```python
from build123d import *

# Parameters (mm, degrees)
CYLINDER002_R           = 2
CYLINDER002_DEPTH       = 10
CYLINDER002_PITCH_ANGLE = 90
CYLINDER003_R           = 2
CYLINDER003_DEPTH       = 10
CYLINDER003_PITCH_ANGLE = 90
CYLINDER001_R           = 2
CYLINDER001_DEPTH       = 10
CYLINDER001_PITCH_ANGLE = 90
CYLINDER_R              = 2
CYLINDER_DEPTH          = 10
CYLINDER_PITCH_ANGLE    = 90
BOX012_W                = 10
BOX012_H                = 4.3
BOX012_DEPTH            = 13
BOX011_W                = 10
BOX011_H                = 1.8
BOX011_DEPTH            = 13
BOX007_W                = 10
BOX007_H                = 1.8
BOX007_DEPTH            = 13
BOX009_W                = 10
BOX009_H                = 4.3
BOX009_DEPTH            = 13
BOX008_W                = 10
BOX008_H                = 4.3
BOX008_DEPTH            = 13
BOX010_W                = 10
BOX010_H                = 1.8
BOX010_DEPTH            = 13
BOX006_W                = 10
BOX006_H                = 4.3
BOX006_DEPTH            = 13
BOX005_W                = 10
BOX005_H                = 1.8
BOX005_DEPTH            = 13
BOX002_W                = 10
BOX002_H                = 25
BOX002_DEPTH            = 77.4
BOX004_W                = 10
BOX004_H                = 25
BOX004_DEPTH            = 77.4
BOX001_W                = 10
BOX001_H                = 25
BOX001_DEPTH            = 77.4
BOX003_W                = 10
BOX003_H                = 25
BOX003_DEPTH            = 77.4
BOX_W                   = 2.3
BOX_H                   = 164.6
BOX_DEPTH               = 256.2
FILLET_R                = 30
FILLET001_R             = 30
FILLET002_R             = 30
FILLET003_R             = 30


with BuildPart() as cilindro002:
    # Cylinder002 → Cylinder002 (new body)
    with BuildSketch(Plane.XY):
        Circle(CYLINDER002_R)
    extrude(amount=CYLINDER002_DEPTH)


with BuildPart() as cilindro002_1:
    # Cylinder002 pitch: moved
    add(cilindro002.part.rotate(Axis((0, 0, 0), (0, 1, 0)), CYLINDER002_PITCH_ANGLE))


with BuildPart() as cilindro002_2:
    # Cylinder002 placement: moved
    add(cilindro002_1.part.moved(Location((-2, 28, 248))))


with BuildPart() as cilindro003:
    # Cylinder003 → Cylinder003 (new body)
    with BuildSketch(Plane.XY):
        Circle(CYLINDER003_R)
    extrude(amount=CYLINDER003_DEPTH)


with BuildPart() as cilindro003_1:
    # Cylinder003 pitch: moved
    add(cilindro003.part.rotate(Axis((0, 0, 0), (0, 1, 0)), CYLINDER003_PITCH_ANGLE))


with BuildPart() as cilindro003_2:
    # Cylinder003 placement: moved
    add(cilindro003_1.part.moved(Location((-2, 142, 248))))


with BuildPart() as cilindro001:
    # Cylinder001 → Cylinder001 (new body)
    with BuildSketch(Plane.XY):
        Circle(CYLINDER001_R)
    extrude(amount=CYLINDER001_DEPTH)


with BuildPart() as cilindro001_1:
    # Cylinder001 pitch: moved
    add(cilindro001.part.rotate(Axis((0, 0, 0), (0, 1, 0)), CYLINDER001_PITCH_ANGLE))


with BuildPart() as cilindro001_2:
    # Cylinder001 placement: moved
    add(cilindro001_1.part.moved(Location((-1, 142, 8))))


with BuildPart() as cilindro:
    # Cylinder → Cylinder (new body)
    with BuildSketch(Plane.XY):
        Circle(CYLINDER_R)
    extrude(amount=CYLINDER_DEPTH)


with BuildPart() as cilindro_1:
    # Cylinder pitch: moved
    add(cilindro.part.rotate(Axis((0, 0, 0), (0, 1, 0)), CYLINDER_PITCH_ANGLE))


with BuildPart() as cilindro_2:
    # Cylinder placement: moved
    add(cilindro_1.part.moved(Location((-2, 28, 8))))


with BuildPart() as cubo012:
    # Box012 → Box012 (new body)
    with BuildSketch(Plane(origin=(-2, 115.2, 160), x_dir=(1, 0, 0), z_dir=(0, 0, 1))):
        with Locations((5, 2.15)):
            Rectangle(BOX012_W, BOX012_H)
    extrude(amount=BOX012_DEPTH)


with BuildPart() as cubo011:
    # Box011 → Box011 (new body)
    with BuildSketch(Plane(origin=(-2, 138.2, 160), x_dir=(1, 0, 0), z_dir=(0, 0, 1))):
        with Locations((5, 0.9)):
            Rectangle(BOX011_W, BOX011_H)
    extrude(amount=BOX011_DEPTH)


with BuildPart() as cubo007:
    # Box007 → Box007 (new body)
    with BuildSketch(Plane(origin=(-2, 138.2, 82.4), x_dir=(1, 0, 0), z_dir=(0, 0, 1))):
        with Locations((5, 0.9)):
            Rectangle(BOX007_W, BOX007_H)
    extrude(amount=BOX007_DEPTH)


with BuildPart() as cubo009:
    # Box009 → Box009 (new body)
    with BuildSketch(Plane(origin=(-2, 115.2, 82.4), x_dir=(1, 0, 0), z_dir=(0, 0, 1))):
        with Locations((5, 2.15)):
            Rectangle(BOX009_W, BOX009_H)
    extrude(amount=BOX009_DEPTH)


with BuildPart() as cubo008:
    # Box008 → Box008 (new body)
    with BuildSketch(Plane(origin=(0, 45.7, 160), x_dir=(1, 0, 0), z_dir=(0, 0, 1))):
        with Locations((5, 2.15)):
            Rectangle(BOX008_W, BOX008_H)
    extrude(amount=BOX008_DEPTH)


with BuildPart() as cubo010:
    # Box010 → Box010 (new body)
    with BuildSketch(Plane(origin=(-2, 25, 160), x_dir=(1, 0, 0), z_dir=(0, 0, 1))):
        with Locations((5, 0.9)):
            Rectangle(BOX010_W, BOX010_H)
    extrude(amount=BOX010_DEPTH)


with BuildPart() as cubo006:
    # Box006 → Box006 (new body)
    with BuildSketch(Plane(origin=(0, 45.7, 82.4), x_dir=(1, 0, 0), z_dir=(0, 0, 1))):
        with Locations((5, 2.15)):
            Rectangle(BOX006_W, BOX006_H)
    extrude(amount=BOX006_DEPTH)


with BuildPart() as cubo005:
    # Box005 → Box005 (new body)
    with BuildSketch(Plane(origin=(-2, 25, 82.4), x_dir=(1, 0, 0), z_dir=(0, 0, 1))):
        with Locations((5, 0.9)):
            Rectangle(BOX005_W, BOX005_H)
    extrude(amount=BOX005_DEPTH)


with BuildPart() as cubo002:
    # Box002 → Box002 (new body)
    with BuildSketch(Plane.XY.offset(145)):
        with Locations((5, 12.5)):
            Rectangle(BOX002_W, BOX002_H)
    extrude(amount=BOX002_DEPTH)


with BuildPart() as cubo004:
    # Box004 → Box004 (new body)
    with BuildSketch(Plane(origin=(0, 140, 145), x_dir=(1, 0, 0), z_dir=(0, 0, 1))):
        with Locations((5, 12.5)):
            Rectangle(BOX004_W, BOX004_H)
    extrude(amount=BOX004_DEPTH)


with BuildPart() as cubo001:
    # Box001 → Box001 (new body)
    with BuildSketch(Plane.XY.offset(33)):
        with Locations((5, 12.5)):
            Rectangle(BOX001_W, BOX001_H)
    extrude(amount=BOX001_DEPTH)


with BuildPart() as cubo003:
    # Box003 → Box003 (new body)
    with BuildSketch(Plane(origin=(0, 140, 33), x_dir=(1, 0, 0), z_dir=(0, 0, 1))):
        with Locations((5, 12.5)):
            Rectangle(BOX003_W, BOX003_H)
    extrude(amount=BOX003_DEPTH)


with BuildPart() as cut015:
    # Box → Box (new body)
    with BuildSketch(Plane.XY):
        with Locations((1.15, 82.3)):
            Rectangle(BOX_W, BOX_H)
    extrude(amount=BOX_DEPTH)

    # Cut: cut Cubo003
    add(cubo003.part, mode=Mode.SUBTRACT)

    # Cut001: cut Cubo001
    add(cubo001.part, mode=Mode.SUBTRACT)

    # Cut002: cut Cubo004
    add(cubo004.part, mode=Mode.SUBTRACT)

    # Cut003: cut Cubo002
    add(cubo002.part, mode=Mode.SUBTRACT)

    # Fillet
    fillet_edges = [cut015.edges().sort_by_distance(p)[0] for p in [
        (1.15, 0, 0),
    ]]
    fillet(fillet_edges, radius=FILLET_R)

    # Fillet001
    fillet001_edges = [cut015.edges().sort_by_distance(p)[0] for p in [
        (1.15, 164.6, 0),
    ]]
    fillet(fillet001_edges, radius=FILLET001_R)

    # Fillet002
    fillet002_edges = [cut015.edges().sort_by_distance(p)[0] for p in [
        (1.15, 164.6, 256.2),
    ]]
    fillet(fillet002_edges, radius=FILLET002_R)

    # Fillet003
    fillet003_edges = [cut015.edges().sort_by_distance(p)[0] for p in [
        (1.15, 0, 256.2),
    ]]
    fillet(fillet003_edges, radius=FILLET003_R)

    # Cut004: cut Cubo005
    add(cubo005.part, mode=Mode.SUBTRACT)

    # Cut005: cut Cubo006
    add(cubo006.part, mode=Mode.SUBTRACT)

    # Cut006: cut Cubo010
    add(cubo010.part, mode=Mode.SUBTRACT)

    # Cut007: cut Cubo008
    add(cubo008.part, mode=Mode.SUBTRACT)

    # Cut008: cut Cubo009
    add(cubo009.part, mode=Mode.SUBTRACT)

    # Cut009: cut Cubo007
    add(cubo007.part, mode=Mode.SUBTRACT)

    # Cut010: cut Cubo011
    add(cubo011.part, mode=Mode.SUBTRACT)

    # Cut011: cut Cubo012
    add(cubo012.part, mode=Mode.SUBTRACT)

    # Cut012: cut Cilindro
    add(cilindro_2.part, mode=Mode.SUBTRACT)

    # Cut013: cut Cilindro001
    add(cilindro001_2.part, mode=Mode.SUBTRACT)

    # Cut014: cut Cilindro003
    add(cilindro003_2.part, mode=Mode.SUBTRACT)

    # Cut015: cut Cilindro002
    add(cilindro002_2.part, mode=Mode.SUBTRACT)


solid = cut015.part
```
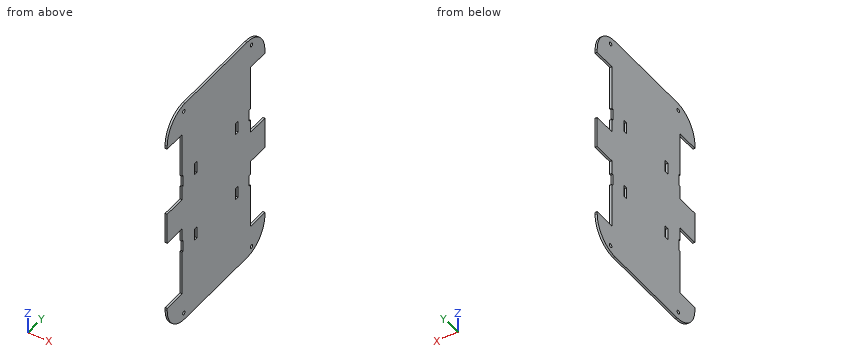
The listing builds one solid part. Answer for the finished solid, in the listing's coordinates (mm). Round coordinates to 2 decimals unless told otherwise and drop trailing zeros. Write each loop counter-clockwise with the first axis right and the second up, starting at its lowest first coordinate (ties: lowest second). Pieces come first, ordered by that corner, then holes. Notation, with made-up numbers: (53, -2.75) -> (73, -2.75) arc R21 cw to (73, 23.25) -> close; hole circle Ø11 at (13.5, 10). An arc over 180 degrees is marked (long way). Answer as a JSON object with one key per item and string values. Group by question number.
Q1. Section D-D (z = 46) is taken. Write down the section's boundary in (x, y).
Q2. Section C-C (x = 0.5) is taken. Count the separate pieces of the cut face and the enclosed holes in it, plus the area to 3 significant figures.
Q3. Section B-B (y = 11) is taken. Write down the section's boundary in (x, z).
Q4. Section A-A (z = 166) is taken. Write down the section's boundary in (x, y), plus the area to 3 significant figures.
Q5. Each of these flat-tipped pins is pushed along its axis until it touches: pin 1 Ø1.2 at (x, z) = (1, 167.5) entering from -Y; pin 2 Ø1.2 at (x, z) = (1, 100) entering from -Y; pin 3 Ø1.2 at (x, z) = (1, 169.5) entering from +Y. Where does it stop, or does it pass through?
Q6. Straight lines are drawn through the part: line 1 along Z through (x, y) = (1.4, 46.5); line 2 along Z through (x, y) = (1.7, 142); line 3 along Z through (x, y) = (1.05, 142.5). For each, find the intervals that lie inside material, in ascending order.
Check values:
{
 "1": {"outline": "(0, 25) -> (2.3, 25) -> (2.3, 140) -> (0, 140) -> close"},
 "2": {"separate pieces": "1", "enclosed holes": "8", "area": "33,400 mm^2"},
 "3": {"outline": "(0, 6.78) -> (2.3, 6.78) -> (2.3, 33) -> (0, 33) -> close; (0, 110.4) -> (2.3, 110.4) -> (2.3, 145) -> (0, 145) -> close; (0, 222.4) -> (2.3, 222.4) -> (2.3, 249.42) -> (0, 249.42) -> close"},
 "4": {"outline": "(0, 26.8) -> (2.3, 26.8) -> (2.3, 45.7) -> (0, 45.7) -> close; (0, 50) -> (2.3, 50) -> (2.3, 115.2) -> (0, 115.2) -> close; (0, 119.5) -> (2.3, 119.5) -> (2.3, 138.2) -> (0, 138.2) -> close", "area": "236 mm^2"},
 "5": {"pin 1": "y = 26.8", "pin 2": "y = 25", "pin 3": "y = 138.2"},
 "6": {"line 1": "0 to 82.4, 95.4 to 160, 173 to 256.2", "line 2": "0.93 to 6, 10 to 33, 110.4 to 145, 222.4 to 246, 250 to 255.27", "line 3": "1.06 to 6.06, 9.94 to 33, 110.4 to 145, 222.4 to 246.06, 249.94 to 255.14"}
}
